The listing builds one solid part. Answer for the finished solid, in the listing's coordinates (mm). Face numbers are marked on the shaded views. A direction names the side the tool comes from. Round coordinates to 2 decimals unless told otherwise and drop trailing zeros. Order: outer loops, then holes, each group sorted by start corner. A loop starts at its lowest first (then second) coordinate and runs counter-clockwise, first axis right, second up. Notation, with made-up numbers: (67, -25.75) - (72, -25.75) arc R20 cw to (72, -15.75) - close; hole circle Ø3 at (74.5, -28). An arc over 180 degrees is marked (long way). Use CSV: the item, a comma, the result in double quotes. Start each with the question number.
Item 1: Find section A-A, the plane z = 0. Give the vertices of the cut face in (x, y), plus the area to 3 significant figures.
Item 2: Straight lines are drawn through the part: line 1 along Y through (x, z) = (1.5, -33); line 2 along Z through (x, y) = (8.5, 35); line 3 along Y through (x, z) = (7, -37.5). For each, find the intervals that lie inside material, in ascending order. Write a range as [from, to].
Item 3: Determine the mould class of the marked faces 1, 2 and 3 for opening direction Y: +Y half, -Y half, draft (parallel to the pull), parting line (faces both ways), or undercut.
Item 4: For the marked faces 4, 5, 6 and 7, determine the directions among +Z, -Z, +X, -X, +Y, -Y from which every point of the face is accessible in a straight line to the end or side of a thin tool.
Item 5: Flat-ended cylindrical pins translate along their axes: P1, Ø15, axis at y = 3.5, z = -6.5, coming from the +X side; P2, Ø1.3, axis at y = 0, z = 12, coming from the -X side; P3, Ø2, axis at x = 3, z = -3, coming from the -Y side; P4, Ø3.5, axis at y = 8.49, z = 8.49, coming from the -X side. Find the tip coordinate at first contact, or state that the pin passes through.
Item 6: Find section C-C, the plane x = 1.5. Count the separate pieces of the cut face and the enclosed holes in it, plus the area to 3 significant figures.
```python
from build123d import *

# Parameters (mm, degrees)
TOOTHCUT_DEPTH     = 65.761099435
TEETHCUTS_COUNT    = 16
TEETHCUTS_ANGLE    = 337.5
BORSKE_R           = 6
BORE_DEPTH         = 50.0000508
SKETCH1_R          = 1.05
CUT_EXTRUDE1_DEPTH = 120


with BuildPart() as part:
    # BasProSke → Base-Revolve (revolve)
    with BuildSketch(Plane(origin=(0, 0, 0), x_dir=(1, 0, 0), z_dir=(0, 1, 0)), mode=Mode.PRIVATE) as base_revolve_sk:
        Polygon((0, 0), (0, 45), (12, 45), (12, 15), (5.5, 15), (5.5, 6), (4, 6), (4, 0), align=None)
    revolve(base_revolve_sk.sketch.rotate(Axis((-10, 0, 0), (1, 0, 0)), 180), axis=Axis((-10, 0, 0), (1, 0, 0)))

    # TooCutSke → ToothCut (cut, through all)
    with BuildSketch(Plane(origin=(0, 0, 0), x_dir=(0, 0, -1), z_dir=(1, 0, 0))):
        with BuildLine():
            ThreePointArc((2.585211293, 33.64983928), (0, 33.749), (-2.585211293, 33.64983928))
            ThreePointArc((-2.585211293, 33.64983928), (-4.077113604, 39.496303475), (-7.62816215, 44.37451732))
            ThreePointArc((-7.62816215, 44.37451732), (0, 45.0254), (7.62816215, 44.37451732))
            ThreePointArc((7.62816215, 44.37451732), (4.077113604, 39.496303475), (2.585211293, 33.64983928))
        make_face()
    toothcut = extrude(amount=TOOTHCUT_DEPTH, mode=Mode.SUBTRACT)

    # TeethCuts: ToothCut ×16 about axis
    teethcuts_axis = Axis((-10, 0, 0), (1, 0, 0))
    for i in range(1, TEETHCUTS_COUNT):
        add(toothcut.rotate(teethcuts_axis, i * TEETHCUTS_ANGLE / (TEETHCUTS_COUNT - 1)), mode=Mode.SUBTRACT)

    # BorSke → Bore (cut, symmetric)
    with BuildSketch(Plane(origin=(0, 0, 0), x_dir=(0, 0, -1), z_dir=(1, 0, 0))):
        with Locations(Location((0, 0, 0), (0, 0, 180))):
            Circle(BORSKE_R)
    extrude(amount=BORE_DEPTH, both=True, mode=Mode.SUBTRACT)

    # Sketch1 → Cut-Extrude1 (cut)
    with BuildSketch(Plane(origin=(12, 0, 0), x_dir=(0, 0, -1), z_dir=(1, 0, 0))):
        with Locations((0, 12)):
            Circle(SKETCH1_R)
        with Locations((8.485281374, 8.485281374)):
            Circle(SKETCH1_R)
        with Locations((12, 0)):
            Circle(SKETCH1_R)
        with Locations((8.485281374, -8.485281374)):
            Circle(SKETCH1_R)
        with Locations((0, -12)):
            Circle(SKETCH1_R)
        with Locations((-8.485281374, -8.485281374)):
            Circle(SKETCH1_R)
        with Locations((-12, 0)):
            Circle(SKETCH1_R)
        with Locations((-8.485281374, 8.485281374)):
            Circle(SKETCH1_R)
    extrude(amount=-CUT_EXTRUDE1_DEPTH, mode=Mode.SUBTRACT)


solid = part.part
```
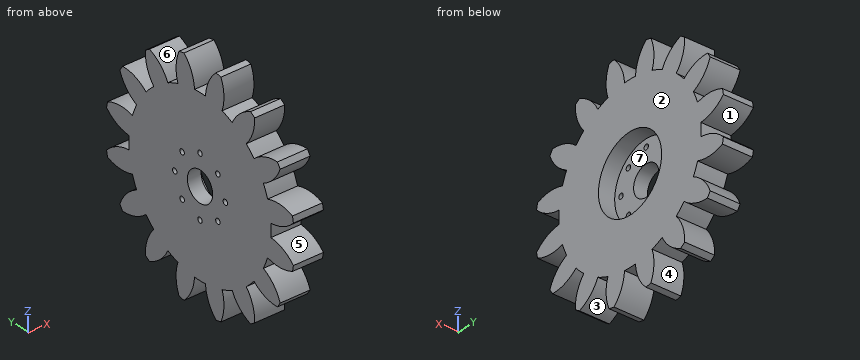
Worked out:
1,outline,"(0, -33.75) - (12, -33.75) - (12, -15) - (5.5, -15) - (5.5, -13.05) - (0, -13.05) - close; (0, -10.95) - (5.5, -10.95) - (5.5, -6) - (0, -6) - close; (0, 6) - (5.5, 6) - (5.5, 10.95) - (0, 10.95) - close; (0, 13.05) - (5.5, 13.05) - (5.5, 15) - (12, 15) - (12, 33.75) - (0, 33.75) - close"
1,area,"526 mm²"
2,line 1,"y = [-25.66, -17.08], [-10.78, 10.78], [17.08, 25.66]"
2,line 2,"z = [-25.94, -18.96], [-11.2, -2.72], [2.72, 11.2], [18.96, 25.94]"
2,line 3,"y = [-24.87, -22.68], [-11.36, -3.3], [3.3, 11.36], [22.68, 24.87]"
3,face 1,"+Y half"
3,face 2,"draft"
3,face 3,"undercut"
4,face 4,"+X, -X"
4,face 5,"+X, -X, -Y"
4,face 6,"+Z, +X, -X"
4,face 7,"+X"
5,P1,"stops at x = 5.5"
5,P2,"passes through"
5,P3,"stops at y = -39.33"
5,P4,"stops at x = 0"
6,separate pieces,"1"
6,enclosed holes,"9"
6,area,"4,660 mm²"
